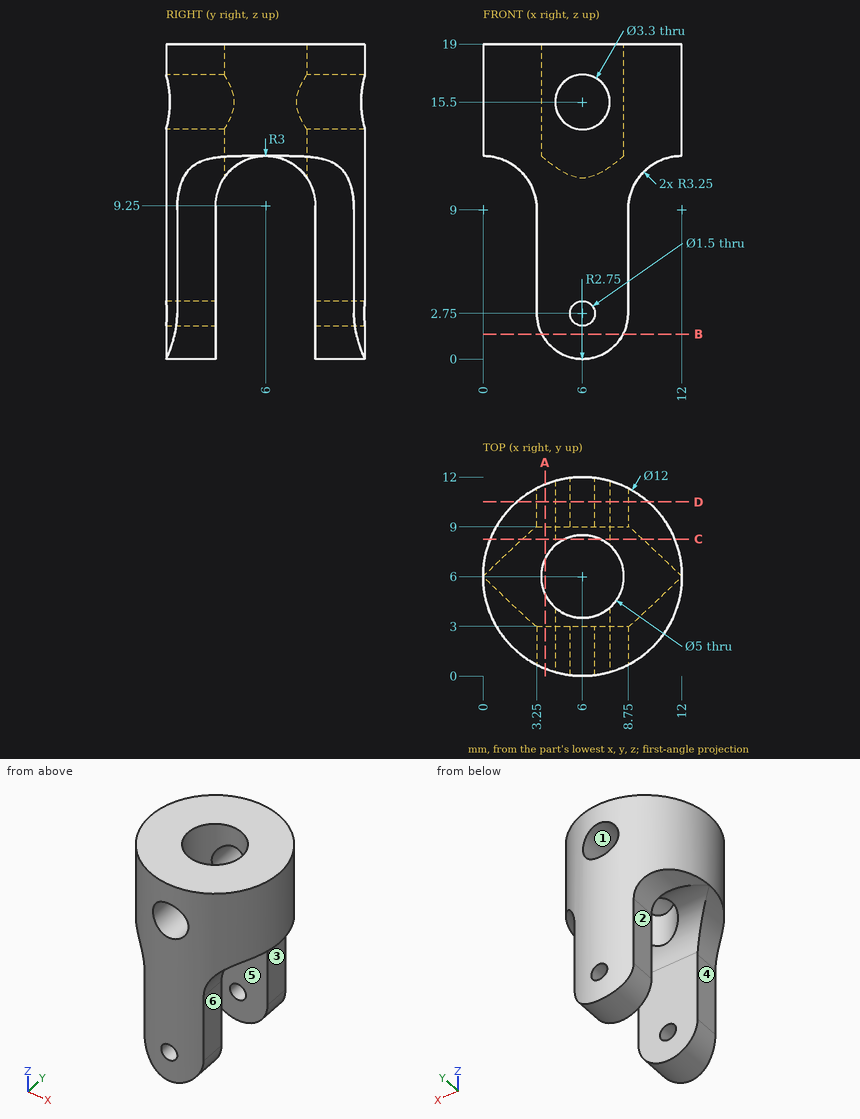
Check sheet for the drawn part. Datum: minimum x, y, z corner. Units: mm. A direction names the side the tool comes from. Give positions to 0.01 mm unless a question says otherwise; leave off trailing zeros. Order: outer loops, then holes, each group sorted by start corner. A loop starts at its lowest first (then second) coordinate and runs counter-clockwise, first axis right, second up. Notation, with made-up numbers: (7, 17.25) -> (25, 17.25) arc R12 cw to (25, 25.25) -> close; hole circle Ø10 at (73.5, 84). An arc over 180 degrees is marked (long way). One line per item, written item: value.
(1) Sectioned sample at A-A on x = 3.75. Record the cut outline in (y, z), then the cut area to 3 significant figures.
Final values:
outline: (0.44, 1.17) -> (3, 1.17) -> (3, 9.25) arc R3 cw to (4.91, 12.05) -> (4.91, 19) -> (0.44, 19) -> close; (7.09, 12.05) arc R3 cw to (9, 9.25) -> (9, 1.17) -> (11.56, 1.17) -> (11.56, 19) -> (7.09, 19) -> close
area: 121 mm^2
(2) Sectioned sample at B-B on z = 1.5. Record the cut outline in (x, y), then the cut area to 3 significant figures.
Final values:
outline: (3.55, 0.52) arc R6 ccw to (8.45, 0.52) -> (8.45, 3) -> (3.55, 3) -> close; (3.55, 9) -> (8.45, 9) -> (8.45, 11.48) arc R6 ccw to (3.55, 11.48) -> close
area: 27.7 mm^2
(3) Sectioned sample at D-D on y = 10.5. Record the cut outline in (x, z).
Final values:
outline: (2.03, 11.54) arc R3.25 cw to (3.25, 9) -> (3.25, 2.75) arc R2.75 ccw to (8.75, 2.75) -> (8.75, 9) arc R3.25 cw to (9.97, 11.54) -> (9.97, 19) -> (2.03, 19) -> close; hole circle Ø3.3 at (6, 15.5); hole circle Ø1.5 at (6, 2.75)
(4) Sectioned sample at C-C on y = 8.25. Record the cut outline in (x, z).
Final values:
outline: (0.44, 12.22) arc R3.25 cw to (2.36, 11.23) -> (4.91, 11.23) -> (4.91, 14.26) arc R1.65 cw to (4.91, 16.74) -> (4.91, 19) -> (0.44, 19) -> close; (7.09, 11.23) -> (9.64, 11.23) arc R3.25 cw to (11.56, 12.22) -> (11.56, 19) -> (7.09, 19) -> (7.09, 16.74) arc R1.65 cw to (7.09, 14.26) -> close
(5) Gauge pin test, flat ends, axial feed: pin 1 (0.7 mm diameter, centred on y = 1.5, z = 4.5, fed in from -X); pin 2 (5.5 mm diameter, centred on x = 6, z = 15.5, fed in from -Y); pin 3 (1.2 mm diameter, centred on y = 2, z = 5, fed in from +X); pin 4 (1.5 mm diameter, centred on x = 9, z = 4.5, fed in from -Y). Record the tip position at first contact, or that the pin passes through.
Final values:
pin 1: x = 3.25
pin 2: y = 0
pin 3: x = 8.75
pin 4: y = 0.44
(6) Tool access check on the marked faces 4, 5 and 6. Record the directions out of +Z, -Z, +X, -X, +Y, -Y that give a thin tool (end or side, any length) a straight path to the whole face; none if there is none.
Final values:
face 4: -Z, -X, +Y, -Y
face 5: -Z, +X, -X
face 6: -Z, +X, +Y, -Y
(7) Draft check along X on the marked faces 1, 2 and 3. Enter one of: pulls with the +X half, pulls with the -X half, needs draft (parallel to the pull), parting line crosses it, or undercut.
Final values:
face 1: undercut
face 2: pulls with the -X half
face 3: pulls with the +X half
(8) Scan lines: line 1 along Z through (x, y) = (6, 10.75); line 2 along Y through (x, z) = (6, 17.25); line 3 along Z through (x, y) = (8, 8.5). Record each from-to range of solid material in increasing order. Write a range as [from, to].
Final values:
line 1: [0, 2], [3.5, 13.85], [17.15, 19]
line 2: [0, 3.5], [8.5, 12]
line 3: [10.91, 19]
